Check sheet for the drawn part. Datum: minimum x, y, z corner. Units: mm. Give positions to 0.01 mm unless a question says otherwise; leave off trailing zeros. Write each loop counter-clockwise with the first axis right and the second up, starting at its lowest first coordinate (ties: lowest second). Pieces come first, ordered by that corner, then holes. Notation, with made-up numbers: M 22.5,47 L 62.5,47 A23 ccw 62.5,77 Z; hole C 43,47 d4. An arc over 180 degrees is marked long. Write item = value, one per line.
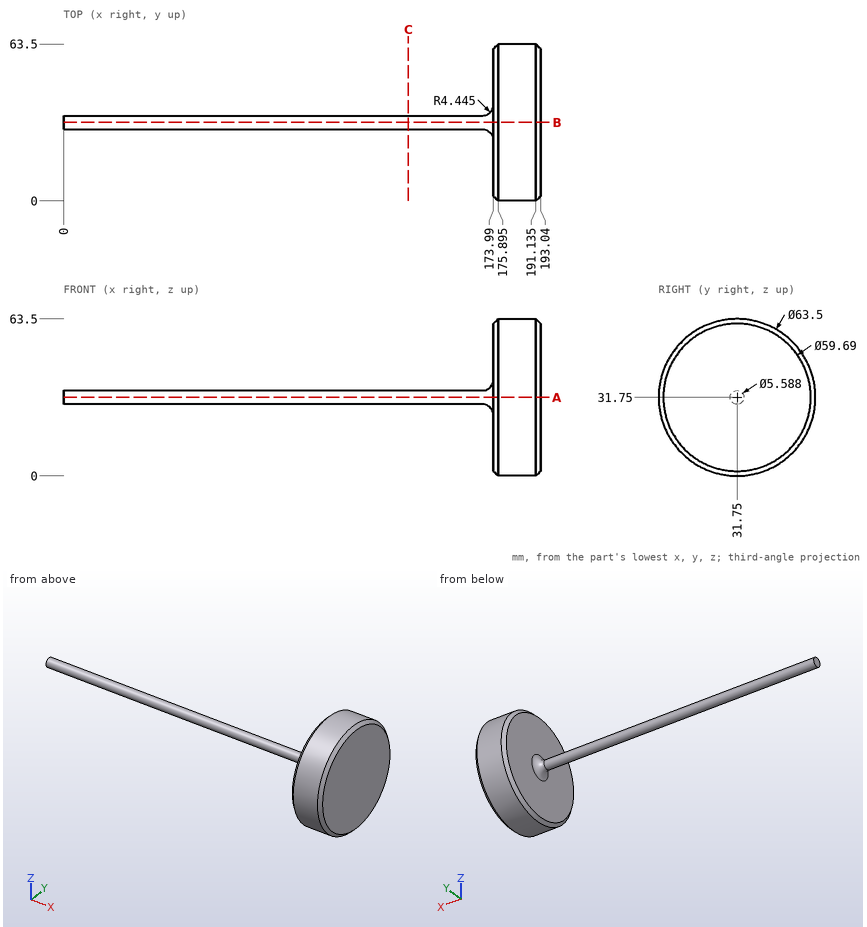
1) Cross-section at C-C on x = 139.5. Record the boundary of the cut face in (y, z), plus the area to 3 significant figures.
From the geometry:
outline = C 31.75,31.75 d5.59
area = 24.5 mm^2
2) Material ranges on probe 1 along X at (y, z) = (9.5, 33); probe 2 along Z at (x, y) = (102, 32); probe 3 along Z at (x, y) = (184, 42.5), recorded low to high. Write a range as from..to.
From the geometry:
probe_1 = 173.99..193.04
probe_2 = 28.97..34.53
probe_3 = 1.88..61.62
3) Depth check by flat-ended pin: P1, Ø1.5, axis at x = 135, y = 33.5, coming from the -Z side; P2, Ø10, axis at x = 101, y = 26, coming from the +Z side; P3, Ø8, axis at x = 133, y = 35, coming from the +Z side. Enter the tip coordinate at first touch or a pass-through.
From the geometry:
P1 = 29.14
P2 = 34.44
P3 = 34.54
4) Cross-section at A-A on z = 31.75. Record the boundary of the cut face in (x, y) (3 decimals).
From the geometry:
outline = M 0,28.956 L 169.545,28.956 A4.445 cw 173.99,24.511 L 173.99,1.905 L 175.895,0 L 191.135,0 L 193.04,1.905 L 193.04,61.595 L 191.135,63.5 L 175.895,63.5 L 173.99,61.595 L 173.99,38.989 A4.445 cw 169.545,34.544 L 0,34.544 Z
